```python
from build123d import *

# Parameters (mm, degrees)
SKETCH1_W           = 6.5
SKETCH1_H           = 10
BOSS_EXTRUDE1_DEPTH = 0.75
SKETCH1_3_W         = 0.75
SKETCH1_3_H         = 10
BOSS_EXTRUDE2_DEPTH = 1.75
FILLET1_R           = 0.5


with BuildPart() as part:
    # Sketch1 → Boss-Extrude1 (new body)
    with BuildSketch(Plane.XY):
        Rectangle(SKETCH1_W, SKETCH1_H)
    extrude(amount=BOSS_EXTRUDE1_DEPTH)

    # Sketch1<3> → Boss-Extrude2 (add)
    with BuildSketch(Plane.XY):
        with Locations((3.625, 0)):
            Rectangle(SKETCH1_3_W, SKETCH1_3_H)
        with Locations((-3.625, 0)):
            Rectangle(SKETCH1_3_W, SKETCH1_3_H)
    extrude(amount=BOSS_EXTRUDE2_DEPTH)

    # Fillet1
    fillet1_edges = [part.edges().sort_by_distance(p)[0] for p in [
        (4, 0, 0),
        (-4, 0, 0),
    ]]
    fillet(fillet1_edges, radius=FILLET1_R)


solid = part.part
```
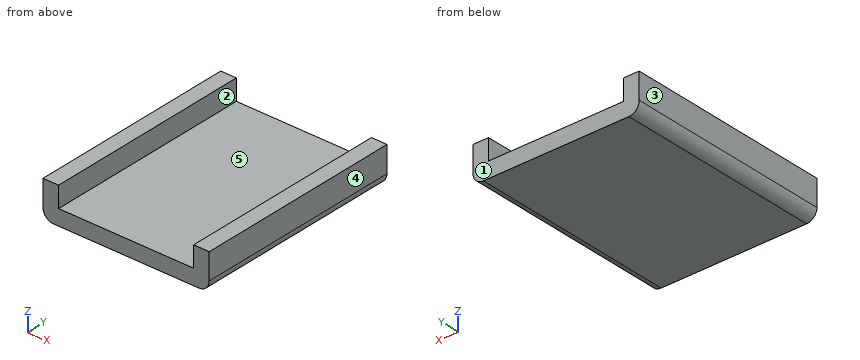
The model under review builds one solid part; all positions refer to its coordinate system, in mm. Face numbers are marked on the shaded views. A direction names the side the tool comes from. Round coordinates to 2 decimals unless told otherwise and drop trailing zeros. Write each loop counter-clockwise with the first axis right and the second up, starting at its lowest first coordinate (ties: lowest second). Pieces come first, ordered by that corner, then holes. Notation, with made-up numbers: (62, 15) - (81, 15) arc R23 ccw to (81, 33) - close; hole circle Ø10 at (-11.5, 31.5). An arc over 180 degrees is marked (long way). One line per question, with ' | ' between items.
Item 1: Add section A-A, the plane z = 1.15. Give the boundary of the cut face in (x, y).
Resolved:
outline: (-4, -5) - (-3.25, -5) - (-3.25, 5) - (-4, 5) - close; (3.25, -5) - (4, -5) - (4, 5) - (3.25, 5) - close
Item 2: For the marked faces 1 and 2, list the 3-axis set-ups (+Z, -Z, +X, -X, +Y, -Y) from which the entire face can be reached by the end or side of a thin tool; tool diameter is ignored.
Resolved:
face 1: +Z, -Z, +X, -X, +Y | face 2: +Z, +Y, -Y
Item 3: Add section C-C, the plane x = 0.5. Give the boundary of the cut face in (y, z).
Resolved:
outline: (-5, 0) - (5, 0) - (5, 0.75) - (-5, 0.75) - close
Item 4: To check wall thickness, follow probe 1 along X at (y, z) = (1.75, 1.25); probe 2 along X at (y, z) = (4, 0.45); probe 3 along Z at (x, y) = (-1, 3.5). State the ranges of each line that lie inside material, in increasing order.
Resolved:
probe 1: x = -4 to -3.25, 3.25 to 4 | probe 2: x = -4 to 4 | probe 3: z = 0 to 0.75
Item 5: For P1, Ø3, axis at x = 1, y = 1.5, coming from the +Z side, flat-tipped, find the tip position at first contact; note if it passes through.
Resolved:
P1: stops at z = 0.75
Item 6: Add section B-B, the plane y = 0. Give the boundary of the cut face in (x, z).
Resolved:
outline: (-4, 0.5) arc R0.5 ccw to (-3.5, 0) - (3.5, 0) arc R0.5 ccw to (4, 0.5) - (4, 1.75) - (3.25, 1.75) - (3.25, 0.75) - (-3.25, 0.75) - (-3.25, 1.75) - (-4, 1.75) - close
Item 7: The part is to be moulded in two halves that separate along X. For the marked faces 3, 4 and 5, say which applies: pulls with the +X half, pulls with the -X half, needs draft (parallel to the pull), parting line crosses it, or undercut.
Resolved:
face 3: pulls with the -X half | face 4: pulls with the +X half | face 5: undercut
Item 8: Add section D-D, the plane z = 0.2. Give the boundary of the cut face in (x, y).
Resolved:
outline: (-3.9, -5) - (3.9, -5) - (3.9, 5) - (-3.9, 5) - close
